from build123d import *

# Parameters (mm, degrees)
F0_W          = 34
F0_H          = 12
F1_DEPTH      = 15
F2_W          = 26
F2_H          = 3.8571179805
F3_DEPTH      = 25
F5_DEPTH      = 6
F5_DEPTH_BACK = 6
F6_R          = 2
F7_DEPTH      = 25
F9_DEPTH      = 1.75
F9_DEPTH_BACK = 1.75
F10_R         = 5


with BuildPart() as f1:
    # F0 (on Front) → F1 (new body)
    with BuildSketch(Plane.XZ):
        Rectangle(F0_W, F0_H)
    extrude(amount=F1_DEPTH)

    # F2 (on face) → F3 (cut)
    with BuildSketch(Plane(origin=(0, 0, -6), x_dir=(1, 0, 0), z_dir=(0, 0, -1))):
        with Locations((0, 7.4285589902)):
            Rectangle(F2_W, F2_H)
    extrude(amount=-F3_DEPTH, mode=Mode.SUBTRACT)

    # F4 (on Top) → F5 (join, two sides)
    with BuildSketch(Plane.XY) as f5_sk:
        with BuildLine():
            Line((-17, -15), (-17, -32))
            ThreePointArc((-17, -32), (0, -49), (17, -32))
            Line((17, -32), (17, -15))
            Line((17, -15), (-17, -15))
        make_face()
    extrude(amount=F5_DEPTH)
    extrude(f5_sk.sketch, amount=-F5_DEPTH_BACK)

    # F6 (on face) → F7 (cut)
    with BuildSketch(Plane.XY.offset(6)):
        with Locations((0, -32)):
            Circle(F6_R)
    extrude(amount=-F7_DEPTH, mode=Mode.SUBTRACT)

    # F8 (on Top) → F9 (cut, two sides)
    with BuildSketch(Plane.XY) as f9_sk:
        with BuildLine():
            Line((-17, -13), (-17, -32))
            ThreePointArc((-17, -32), (0, -49), (17, -32))
            Line((17, -32), (17, -13))
            Line((17, -13), (0, -13))
            Line((0, -13), (-17, -13))
        make_face()
    extrude(amount=-F9_DEPTH, mode=Mode.SUBTRACT)
    extrude(f9_sk.sketch, amount=F9_DEPTH_BACK, mode=Mode.SUBTRACT)

    # F10
    f10_edges = [f1.edges().sort_by_distance(p)[0] for p in [
        (-17, 0, 0),
        (17, 0, 0),
    ]]
    fillet(f10_edges, radius=F10_R)


solid = f1.part
Read the model definition and answer for the solid it produces. Units are mm, in the model's axes. A direction names the side the tool comes from. Give positions to 0.01 mm unless a question says otherwise; leave off trailing zeros. Write each loop counter-clockwise with the first axis right and the second up, starting at its lowest first coordinate (ties: lowest second). Pieces come first, ordered by that corner, then holes. Notation, with made-up numbers: (66, 13.25) - (82, 13.25) arc R11 cw to (82, 32.25) - close; hole circle Ø4 at (4, 89). An arc over 180 degrees is marked (long way). Use CSV: the item, a comma, the result in double quotes. Start each with the question number.
(1) Determine the mould class of faces 4 (the flat face through (0, -24, 6)), 5 (the flat face through (0, -5.5, 0)), 6 (the cylindrical face through (-16, -2, 0)) for opening direction X: +X half, -X half, draft (parallel to the pull), parting line (faces both ways), or undercut.
(2) Find section A-A (x = 0). Give the vertices of the cut face in (y, z).
(3) Find section B-B (y = -28.5). Give the vertices of the cut face in (x, z), plus the area to 3 significant figures.
(4) Find section D-D (z = -3.75). Give the vertices of the cut face in (x, y), plus the area to 3 significant figures.
(5) Find section C-C (x = -8). Give the vertices of the cut face in (y, z), plus the area to 3 significant figures.
(6) For faces 1 (the flat face through (0, 0, 0)), 2 (the flat face through (-13, -7, 0)), 3 (the flat face through (0, -13, 0)), determine the directions among +Z, -Z, +X, -X, +Y, -Y from which every point of the face is accessible in a straight line to the end or side of a thin tool.
(7) Given P1, Ø1, axis at x = -0.5, z = 1, coming from the -Y side; P2, Ø3, axis at x = -5, z = 4, coming from the -Y side, each flat-ended and moving along its own axis, determine where each tip first touches the part or whether it passes through.
(8) Consider line 1 along Y through (x, z) = (0, 3.85); line 2 along Y through (x, z) = (4.5, -1.5); line 3 along Z through (x, y) = (-12.5, -15.5). Determine where each line is inside the solid, lowest interval first.
Findings below:
1,face 4,"draft"
1,face 5,"undercut"
1,face 6,"-X half"
2,outline,"(-49, -6) - (-34, -6) - (-34, -1.75) - (-49, -1.75) - close; (-49, 1.75) - (-34, 1.75) - (-34, 6) - (-49, 6) - close; (-30, -6) - (-9.36, -6) - (-9.36, 6) - (-30, 6) - (-30, 1.75) - (-13, 1.75) - (-13, -1.75) - (-30, -1.75) - close; (-5.5, -6) - (0, -6) - (0, 6) - (-5.5, 6) - close"
3,outline,"(-17, -6) - (17, -6) - (17, -1.75) - (-17, -1.75) - close; (-17, 1.75) - (17, 1.75) - (17, 6) - (-17, 6) - close"
3,area,"289 mm2"
4,outline,"(-17, -32) arc R17 ccw to (17, -32) - (17, -5) arc R5 ccw to (12, 0) - (-12, 0) arc R5 ccw to (-17, -5) - close; hole (-13, -9.36) - (13, -9.36) - (13, -5.5) - (-13, -5.5) - close; hole circle Ø4 at (0, -32)"
4,area,"1,420 mm2"
5,outline,"(-47, -6) - (-9.36, -6) - (-9.36, 6) - (-47, 6) - (-47, 1.75) - (-13, 1.75) - (-13, -1.75) - (-47, -1.75) - close; (-5.5, -6) - (0, -6) - (0, 6) - (-5.5, 6) - close"
5,area,"399 mm2"
6,face 1,"+Z, -Z, +X, -X, +Y"
6,face 2,"+Z, -Z"
6,face 3,"+X, -X, -Y"
7,P1,"y = -13"
7,P2,"y = -48.64"
8,line 1,"-49 to -34, -30 to -9.36, -5.5 to 0"
8,line 2,"-13 to -9.36, -5.5 to 0"
8,line 3,"-6 to -1.75, 1.75 to 6"
